from build123d import *

# Parameters (mm, degrees)
SKETCH1_R               = 30
BOSS_EXTRUDE1_DEPTH     = 5
SKETCH2_R               = 9.5
BOSS_EXTRUDE2_DEPTH     = 80
SKETCH3_R               = 17
BOSS_EXTRUDE3_DEPTH     = 38
FILLET1_R               = 8
SKETCH4_W               = 21.418583827
SKETCH4_H               = 30
CUT_EXTRUDE1_DEPTH      = 19
CUT_EXTRUDE2_DEPTH      = 98.628120949
CUT_EXTRUDE2_DEPTH_BACK = 98.628120949
SKETCH8_R               = 7.5
SKETCH9_R               = 14.5
SKETCH9_R_2             = 7.5
BOSS_EXTRUDE4_DEPTH     = 16.5


with BuildPart() as part:
    # Sketch1 → Boss-Extrude1 (new body)
    with BuildSketch(Plane(origin=(0, 0, 0), x_dir=(1, 0, 0), z_dir=(0, 1, 0))):
        with Locations(Location((0, 0, 0), (0, 0, 270))):
            Circle(SKETCH1_R)
    extrude(amount=BOSS_EXTRUDE1_DEPTH)

    # Sketch2 → Boss-Extrude2 (add)
    with BuildSketch(Plane(origin=(0, 5, 0), x_dir=(1, 0, 0), z_dir=(0, 1, 0))):
        with Locations(Location((0, 0, 0), (0, 0, 270))):
            Circle(SKETCH2_R)
    extrude(amount=BOSS_EXTRUDE2_DEPTH)

    # Sketch3 → Boss-Extrude3 (add)
    with BuildSketch(Plane.XZ):
        with Locations(Location((0, 0, 0), (0, 0, 270))):
            Circle(SKETCH3_R)
    extrude(amount=BOSS_EXTRUDE3_DEPTH)

    # Fillet1
    fillet1_edges = [part.edges().sort_by_distance(p)[0] for p in [
        (0, -38, 17),
    ]]
    fillet(fillet1_edges, radius=FILLET1_R)

    # Sketch4 → Cut-Extrude1 (cut, symmetric)
    with BuildSketch(Plane.XY):
        with Locations((-18.209291914, -23)):
            Rectangle(SKETCH4_W, SKETCH4_H)
        with Locations((18.209291914, -23)):
            Rectangle(SKETCH4_W, SKETCH4_H)
    extrude(amount=CUT_EXTRUDE1_DEPTH, both=True, mode=Mode.SUBTRACT)

    # Sketch8 → Cut-Extrude2 (cut, two sides: drawn at the far end of the back side and taken through both)
    with BuildSketch(Plane(origin=(7.5, 0, 0), x_dir=(0, 0, -1), z_dir=(1, 0, 0)).offset(-CUT_EXTRUDE2_DEPTH_BACK)):
        with Locations(Location((0, -23, 0), (0, 0, 180))):
            Circle(SKETCH8_R)
    extrude(amount=CUT_EXTRUDE2_DEPTH + CUT_EXTRUDE2_DEPTH_BACK, mode=Mode.SUBTRACT)

    # Sketch9 → Boss-Extrude4 (add, symmetric)
    with BuildSketch(Plane(origin=(0, 0, 0), x_dir=(0, 0, -1), z_dir=(1, 0, 0))):
        with Locations(Location((0, -23, 0), (0, 0, 180))):
            Circle(SKETCH9_R)
        with Locations((0, -23)):
            Circle(SKETCH9_R_2, mode=Mode.SUBTRACT)
    extrude(amount=BOSS_EXTRUDE4_DEPTH, both=True)


solid = part.part
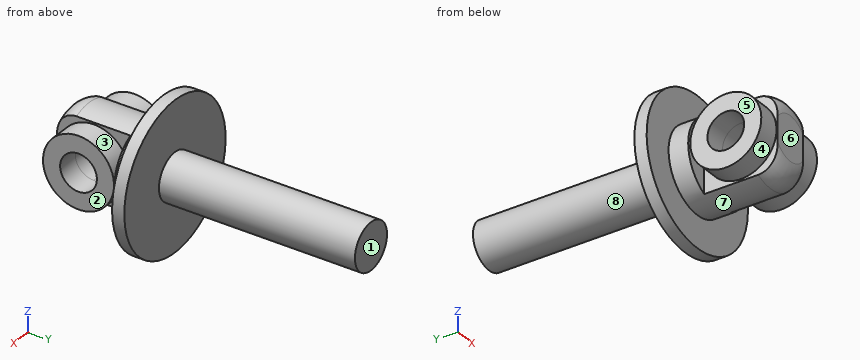
Verification items for the finished model (mm, model axes). Face numbers are marked on the shaded views. A direction names the side the tool comes from. Coordinates: 2 decimals unless noted, no trailing zeros. Order: outer loops, then holes, each group sorted by start corner. A loop starts at its lowest first (then second) coordinate and runs counter-clockwise, first axis right, second up.
1. Set-up check for the marked faces 5, 6, 7 and 8: record each of +Z, -Z, +X, -X, +Y, -Y from which the full face is reachable in a straight line by a thin tool's end or side.
Results found:
face 5: +Z, -Z, -X, -Y
face 6: +Z, -Z, +X, -X, -Y
face 7: none
face 8: +Y
2. Sectioned sample at D-D, the plane x = 0. Record the cut outline in (y, z).
Results found:
outline: (-38, -9) arc R8 ccw to (-30, -17) - (0, -17) - (0, -30) - (5, -30) - (5, -9.5) - (85, -9.5) - (85, 9.5) - (5, 9.5) - (5, 30) - (0, 30) - (0, 17) - (-30, 17) arc R8 ccw to (-38, 9) - close; hole circle Ø15 at (-23, 0)
3. Go/stop test with flat-tipped pins: pin 1 Ø2 at (x, z) = (8.5, -15.5) entering from +Y; pin 2 Ø4.5 at (x, z) = (10, -7) entering from -Y; pin 3 Ø3 at (x, y) = (-0.5, 27) entering from +Z; pin 4 Ø10 at (x, y) = (-4, 6.5) entering from +Z. Record where each tip stops, or that it passes through.
Results found:
pin 1: stops at y = 5
pin 2: stops at y = -36.7
pin 3: stops at z = 9.5
pin 4: stops at z = 30
4. Scan lines: line 1 (Y direction, x = 12.5, z = 0); line 2 (Z direction, x = 14, y = -23); line 3 (Z direction, x = 1, y = -2). Record each from-to range of solid material in increasing order.
Results found:
line 1: y = -37.5 to -30.5, -15.5 to -8.5, -8 to 5
line 2: z = -14.5 to -7.5, 7.5 to 14.5
line 3: z = -16.97 to 16.97
5. Sectioned sample at A-A, the plane x = -13. Record the cut outline in (y, z).
Results found:
outline: circle Ø29 at (-23, 0); (-8, -10.95) - (0, -10.95) - (0, -27.04) - (5, -27.04) - (5, 27.04) - (0, 27.04) - (0, 10.95) - (-8, 10.95) - close; hole circle Ø15 at (-23, 0)
6. Release check for a two-part mould opening along Y. For the marked faces 1, 2, 3 and 4 record: +Y half, -Y half, draft (parallel to the pull), parting line (faces both ways), or undercut.
Results found:
face 1: +Y half
face 2: draft
face 3: undercut
face 4: undercut
7. Sectioned sample at B-B, the plane z = 0. Record the cut outline in (x, y), and give its area (3 significant figures).
Results found:
outline: (-30, 0) - (-17, 0) - (-17, -8) - (-7.5, -8) - (-7.5, -8.5) - (-16.5, -8.5) - (-16.5, -15.5) - (16.5, -15.5) - (16.5, -8.5) - (7.5, -8.5) - (7.5, -8) - (17, -8) - (17, 0) - (30, 0) - (30, 5) - (9.5, 5) - (9.5, 85) - (-9.5, 85) - (-9.5, 5) - (-30, 5) - close; (-16.5, -37.5) - (-7.5, -37.5) - (-7.5, -38) - (7.5, -38) - (7.5, -37.5) - (16.5, -37.5) - (16.5, -30.5) - (-16.5, -30.5) - close
area: 2,570 mm2
8. Sectioned sample at C-C, the plane y = -19.5. Record the cut outline in (x, z), and give its area (3 significant figures).
Results found:
outline: (-16.5, -14.07) - (-7.5, -14.07) - (-7.5, -15.26) arc R17 ccw to (7.5, -15.26) - (7.5, -14.07) - (16.5, -14.07) - (16.5, -6.63) - (-16.5, -6.63) - close; (-16.5, 6.63) - (16.5, 6.63) - (16.5, 14.07) - (7.5, 14.07) - (7.5, 15.26) arc R17 ccw to (-7.5, 15.26) - (-7.5, 14.07) - (-16.5, 14.07) - close
area: 562 mm2
